Study the drawing (mm; zero at the part's minimum x, y, z) and answer. Round coordinates to 2 decimals unless told otherwise and drop trailing zeros. Loops run counter-clockwise (first coordinate to the right, second up) from the corner with the lowest first, then second, coordinate; pieces in that order, holes last. Notation, with made-up numbers: (65.5, 4.5) - (71.5, 4.5) arc R17 cw to (71.5, 17.5) - close; hole circle Ø8 at (60, 4.5). An arc over 180 degrees is marked (long way). One line per item, written item: value.
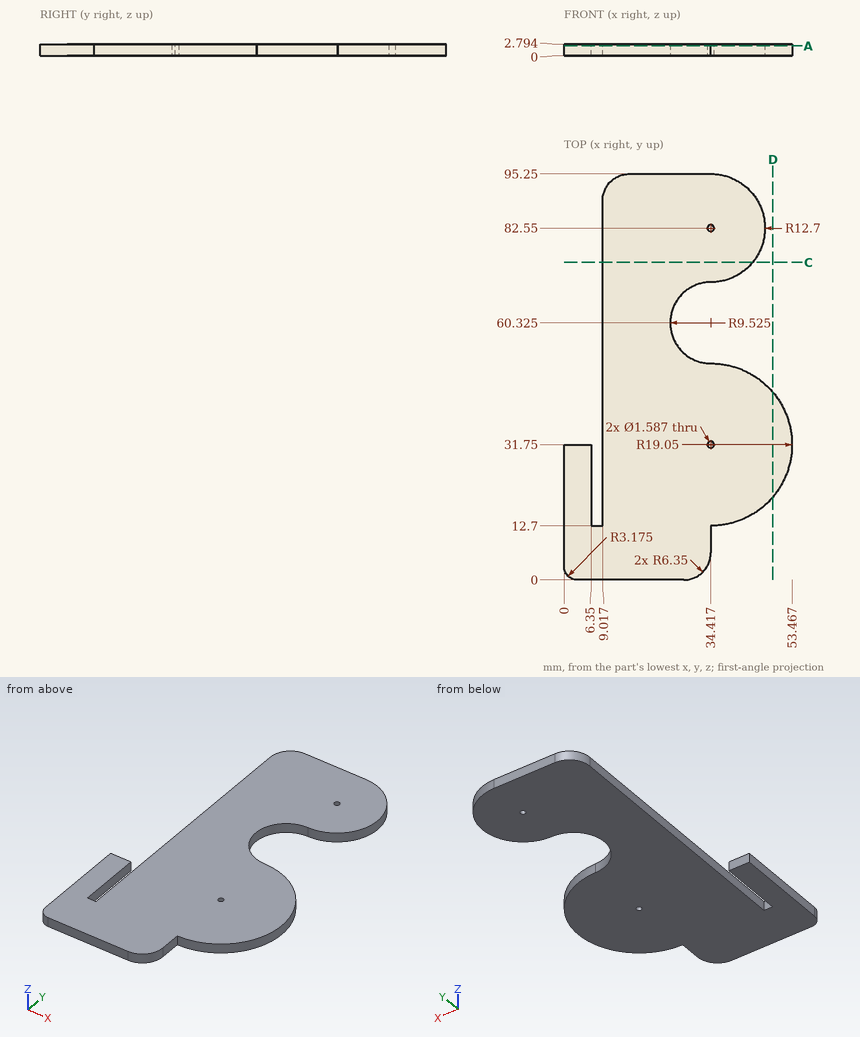
1) Consider L1, parallel to X at y = 82.55, z = 0.7; L2, parallel to Y at x = 43, z = 0.65 (1 decimal); L3, parallel to Y at x = 5.5, z = 2.25. Determine where each line is inside the solid, lowest interval first.
Final values:
L1: 9.02 to 33.62, 35.21 to 47.12
L2: 14.7 to 48.8, 73.2 to 91.9
L3: 0 to 31.75
2) Each of these flat-tipped pins is pushed along its axis until it touches: pin 1 Ø1 at (x, y) = (45.5, 49.5) entering from -Z; pin 2 Ø0.8 at (y, z) = (25, 2) entering from +X; pin 3 Ø0.8 at (x, z) = (8, 1) entering from +Y. Where does it stop, or does it pass through?
Final values:
pin 1: through
pin 2: x = 52.38
pin 3: y = 12.7
3) A cutting plane is placed at D-D on x = 49. Give the vertices of the cut face in (y, z) (1 decimal).
Final values:
outline: (19.5, 0) - (44, 0) - (44, 2.8) - (19.5, 2.8) - close
4) A cutting plane is placed at A-A on z = 2.35. Give the number of separate pieces and of enclosed holes in the cut face, and give its area (3 significant figures).
Final values:
separate pieces: 1
enclosed holes: 2
area: 3,310 mm2
5) A cutting plane is placed at C-C on y = 74.5. Give the vertices of the cut face in (x, z) (1 decimal).
Final values:
outline: (9, 0) - (44.2, 0) - (44.2, 2.8) - (9, 2.8) - close
